Geometry: final body of the model. Coordinates: model frame, mm. A direction names the side the tool comes from. Coordinates: 2 decimals unless noted, no trailing zeros. Loops run counter-clockwise (first coordinate to the right, second up) from the corner with the lowest first, then second, coordinate; pieces in that order, holes last. Notation, with made-up numbers: (72, -4.75) - (124, -4.75) arc R11 ccw to (124, 16.25) - close; hole circle Ø8 at (20, 66.25). An arc over 180 degrees is marked (long way). Return JSON: item names as keys, results as strings.
from build123d import *

# Parameters (mm, degrees)
SKETCH_1_W                  = 41.5
SKETCH_1_H                  = 40
EXTRUDE_1_DEPTH             = 1.5
SKETCH_2_W                  = 1.5
SKETCH_2_H                  = 40
EXTRUDE_2_DEPTH             = 44.5
CUT_EXTRUDE_1_DEPTH         = 1.5
HOLE_WIZARD_3_2_3_2_1_D     = 3.2
HOLE_WIZARD_3_2_3_2_2_D     = 3.2
HOLE_WIZARD_3_2_3_2_2_DEPTH = 1.5
HOLE_WIZARD_3_2_3_2_2_TIP   = 0.96137699
FILLET_1_R                  = 3


with BuildPart() as part:
    # 草图1 → 凸台-拉伸1 (new body)
    with BuildSketch(Plane(origin=(0, 0, 0), x_dir=(1, 0, 0), z_dir=(0, 1, 0))):
        with Locations((20.75, 20)):
            Rectangle(SKETCH_1_W, SKETCH_1_H)
    extrude(amount=EXTRUDE_1_DEPTH)

    # 草图2 → 凸台-拉伸2 (add)
    with BuildSketch(Plane(origin=(0, 1.5, 0), x_dir=(1, 0, 0), z_dir=(0, 1, 0))):
        with Locations((0.75, 20)):
            Rectangle(SKETCH_2_W, SKETCH_2_H)
    extrude(amount=EXTRUDE_2_DEPTH)

    # 草图3 → 切除-拉伸1 (cut)
    with BuildSketch(Plane.ZY):
        with BuildLine():
            Line((-40, 46), (-40, 26))
            ThreePointArc((-40, 26), (-34.142135624, 40.142135624), (-20, 46))
            Line((-20, 46), (-40, 46))
        make_face()
        with BuildLine():
            Line((0, 46), (-20, 46))
            ThreePointArc((-20, 46), (-5.857864376, 40.142135624), (0, 26))
            Line((0, 26), (0, 46))
        make_face()
        with BuildLine():
            Line((-26.5, 19), (-26.5, 33))
            ThreePointArc((-26.5, 33), (-20, 39.5), (-13.5, 33))
            Line((-13.5, 33), (-13.5, 19))
            ThreePointArc((-13.5, 19), (-20, 12.5), (-26.5, 19))
        make_face()
    extrude(amount=-CUT_EXTRUDE_1_DEPTH, mode=Mode.SUBTRACT)

    # Ø3.2 (3.2) 直径孔1 (through all)
    with Locations(Plane.ZY):
        with Locations((-12.25, 39.423393759), (-4.5, 26), (-12.25, 12.576606241), (-27.75, 12.576606241), (-35.5, 26), (-27.75, 39.423393759)):
            Hole(HOLE_WIZARD_3_2_3_2_1_D / 2)

    # Ø3.2 (3.2) 直径孔2
    with Locations(Plane(origin=(0, 0, 0), x_dir=(-1, 0, 0), z_dir=(0, -1, 0))):
        with Locations((-9.5, 31.786000063), (-33.5, 31.786000063), (-33.5, 7.786000063), (-9.5, 7.786000063)):
            Hole(HOLE_WIZARD_3_2_3_2_2_D / 2, depth=HOLE_WIZARD_3_2_3_2_2_DEPTH)
            with Locations((0, 0, -(HOLE_WIZARD_3_2_3_2_2_DEPTH + HOLE_WIZARD_3_2_3_2_2_TIP / 2))):  # 118° drill point
                Cone(0, HOLE_WIZARD_3_2_3_2_2_D / 2, HOLE_WIZARD_3_2_3_2_2_TIP, mode=Mode.SUBTRACT)

    # 圆角1
    fillet_1_edges = [part.edges().sort_by_distance(p)[0] for p in [
        (41.5, 0.75, -40),
        (41.5, 0.75, 0),
    ]]
    fillet(fillet_1_edges, radius=FILLET_1_R)


solid = part.part
Item 1: Section query C-C, the plane z = -22. Return loops of the section in (x, y), and give its area (3 significant figures).
Worked out:
{"outline": "(0, 0) - (41.5, 0) - (41.5, 1.5) - (1.5, 1.5) - (1.5, 12.82) - (0, 12.82) - close; (0, 39.18) - (1.5, 39.18) - (1.5, 45.9) - (0, 45.9) - close", "area": "89.3 mm^2"}
Item 2: Mould query, pull axis Z, two halves, no side actions, for faces 1 (the face through (13, 1, 0)), 2 (the face through (41.5, 1, -20)), 3 (the face through (1, 26, -26.5)). Classes: +Z half, -Z half, draft (parallel to the pull), parting line (faces both ways), or undercut.
Worked out:
{"face 1": "+Z half", "face 2": "draft", "face 3": "undercut"}
Item 3: First-contact query: pin 1 Ø5 at (x, z) = (9.5, -31.786) entering from +Y; pin 2 Ø1.6 at (x, y) = (0.5, 27.5) entering from +Z; pin 3 Ø3 at (y, z) = (26, -35.5) entering from -X; pin 4 Ø4 at (y, z) = (12.58, -27.75) entering from +X. Flat tips, straight axial feed; report the tip coordinate or a pass-through.
Worked out:
{"pin 1": "y = 1.5", "pin 2": "z = -0.01", "pin 3": "through", "pin 4": "x = 1.5"}
Item 4: Section query A-A, the plane x = 33.5. Return loops of the section in (y, z).
Worked out:
{"outline": "(0, -40) - (1.5, -40) - (1.5, -33.39) - (0, -33.39) - close; (0, -30.19) - (1.5, -30.19) - (1.5, -9.39) - (0, -9.39) - close; (0, -6.19) - (1.5, -6.19) - (1.5, 0) - (0, 0) - close"}
Item 5: Reachability of faces 4 (the face through (0.7, 39.5, -20.1)), 5 (the face through (40.64, 0.76, -39.1)), 6 (the face through (1.5, 14, -15)) from +Z, -Z, +X, -X, +Y, -Y: full face, straight path, thin tool, end or side. Return the list, or none.
Worked out:
{"face 4": "+X, -X", "face 5": "-Z, +X, +Y, -Y", "face 6": "+Z, -Z, +X, +Y"}
Item 6: Section query B-B, the plane z = -7. Return loops of the section in (x, y), and give its area (3 significant figures).
Worked out:
{"outline": "(0, 0) - (8.11, 0) - (8.11, 1.5) - (1.5, 1.5) - (1.5, 41.2) - (0, 41.2) - close; (10.89, 0) - (32.11, 0) - (32.11, 1.5) - (10.89, 1.5) - close; (34.89, 0) - (41.5, 0) - (41.5, 1.5) - (34.89, 1.5) - close", "area": "113 mm^2"}
Item 7: Section query D-D, the plane y = 5. Return loops of the section in (x, z).
Worked out:
{"outline": "(0, -40) - (1.5, -40) - (1.5, 0) - (0, 0) - close"}
Item 8: Ray query, probe 1 along Z at (x, y) = (33.5, 0.75); probe 2 along Z at (x, y) = (9, 1); probe 3 along Y at (x, z) = (1.1, -27.75). Return the intervals inside material, ascending. Write a range as from..to.
Worked out:
{"probe 1": "-40..-33.39, -30.19..-9.39, -6.19..0", "probe 2": "-40..-33.31, -30.27..-9.31, -6.27..0", "probe 3": "0..10.98, 14.18..37.82, 41.02..44.44"}
